Work out the finished part from the listing and answer in its coordinate system (mm). Face numbers are marked on the shaded views. A direction names the side the tool comes from. Round coordinates to 2 decimals unless told otherwise and drop trailing zeros. Loops run counter-clockwise (first coordinate to the right, second up) from the corner with the lowest first, then second, coordinate; pieces in that order, holes last. Notation, with made-up numbers: (-15.5, 24.5) - (12.5, 24.5) arc R22 cw to (12.5, 47.5) - close; hole circle Ø1 at (-16, 49.25). An arc over 180 degrees is marked (long way). Return JSON: item names as keys, results as strings.
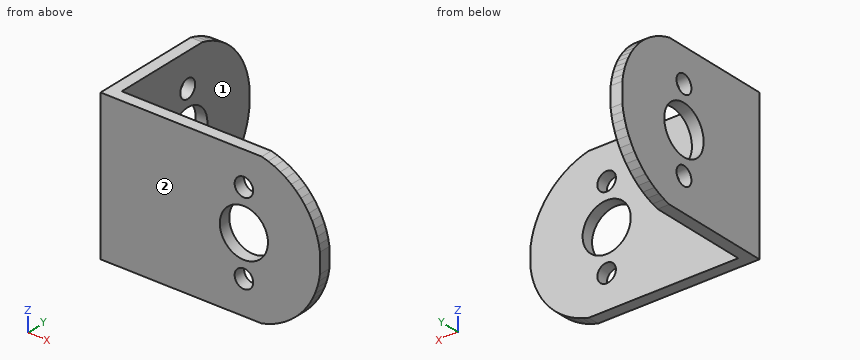
from build123d import *

# Parameters (mm, degrees)
SALIENTE_EXTRUIR1_DEPTH = 2.000000328
CROQUIS2_W              = 2.000000328
CROQUIS2_H              = 25.499995797
SALIENTE_EXTRUIR2_DEPTH = 17.052894691
SALIENTE_EXTRUIR3_DEPTH = 2.000000095
CORTAR_EXTRUIR1_DEPTH   = 92.062133489
CORTAR_EXTRUIR2_DEPTH   = 92.062133489
CORTAR_EXTRUIR3_DEPTH   = 85.413414633
CORTAR_EXTRUIR4_DEPTH   = 85.413414633
CORTAR_EXTRUIR5_DEPTH   = 85.413414633
CORTAR_EXTRUIR6_DEPTH   = 91.256922872
CROQUIS10_R             = 4.160635969
CROQUIS10_R_2           = 1.574242088
CORTAR_EXTRUIR7_DEPTH   = 92.062133489
CROQUIS11_R             = 4.116064073
CROQUIS11_R_2           = 1.582596422
CORTAR_EXTRUIR8_DEPTH   = 86.074229775


with BuildPart() as part:
    # Croquis1 → Saliente-Extruir1 (new body)
    with BuildSketch(Plane(origin=(-18.750000745, 0, 0), x_dir=(0, -1, 0), z_dir=(-1, 0, 0))):
        Polygon((-19.052894786, -77.749997377), (-19.052894786, -52.25000158), (-20.138457417, -52.559908479), (-21.193336695, -52.962061018), (-22.209705785, -53.453475237), (-23.180030286, -54.030507803), (-24.097116664, -54.688870907), (-24.954162538, -55.423695594), (-25.744814426, -56.229524314), (-26.46320872, -57.100389153), (-27.104021981, -58.029823005), (-27.662498876, -59.010945261), (-28.134498745, -60.036472976), (-28.51652354, -61.098802835), (-28.805738315, -62.190063298), (-28.999999166, -63.302159309), (-28.999999166, -66.697835922), (-28.805738315, -67.809939384), (-28.51652354, -68.901196122), (-28.134498745, -69.963529706), (-27.662498876, -70.989057422), (-27.104021981, -71.970179677), (-26.46320872, -72.899609804), (-25.744814426, -73.770478368), (-24.954162538, -74.576310813), (-24.097116664, -75.311124325), (-23.180030286, -75.969494879), (-22.209705785, -76.546527445), (-21.193336695, -77.037930489), (-20.138457417, -77.440083027), align=None)
    extrude(amount=-SALIENTE_EXTRUIR1_DEPTH)

    # Croquis2 → Saliente-Extruir2 (add)
    with BuildSketch(Plane.XZ.offset(-19.052894786)):
        with Locations((-17.750000581, -64.999999479)):
            Rectangle(CROQUIS2_W, CROQUIS2_H)
    extrude(amount=SALIENTE_EXTRUIR2_DEPTH)

    # Croquis3 → Saliente-Extruir3 (add)
    with BuildSketch(Plane.XZ.offset(-2.000000095)):
        Polygon((8.802894503, -77.749997377), (-18.750000745, -77.749997377), (-18.750000745, -52.25000158), (8.802894503, -52.25000158), (9.888458066, -52.559908479), (10.943335481, -52.962061018), (11.959705502, -53.453475237), (12.930030003, -54.030507803), (13.84711545, -54.688870907), (14.704162255, -55.423695594), (15.494815074, -56.229524314), (16.213208437, -57.100389153), (16.854021698, -58.029823005), (17.412498593, -59.010945261), (17.884498462, -60.036472976), (18.266523257, -61.098802835), (18.555738032, -62.190063298), (18.750000745, -63.302159309), (18.750000745, -66.697835922), (18.555738032, -67.809939384), (18.266523257, -68.901196122), (17.884498462, -69.963529706), (17.412498593, -70.989057422), (16.854021698, -71.970179677), (16.213208437, -72.899609804), (15.494815074, -73.770478368), (14.704162255, -74.576310813), (13.84711545, -75.311124325), (12.930030003, -75.969494879), (11.959705502, -76.546527445), (10.943335481, -77.037930489), (9.888458066, -77.440083027), align=None)
    extrude(amount=SALIENTE_EXTRUIR3_DEPTH)

    # Croquis4 → Cortar-Extruir1 (cut, through all)
    with BuildSketch(Plane.ZY.offset(18.750000745)):
        Polygon((-67.884810269, 13.229101896), (-67.402966321, 12.802229263), (-66.858895123, 12.458175421), (-66.266670823, 12.205854058), (-65.641649067, 12.051798403), (-64.999997616, 12.000000104), (-64.358353615, 12.051798403), (-63.733331859, 12.205854058), (-63.141107559, 12.458175421), (-62.597028911, 12.802229263), (-62.115188688, 13.229101896), (-61.708066612, 13.727741316), (-61.386201531, 14.285230078), (-61.157926917, 14.887129888), (-61.029162258, 15.517854132), (-61.003241688, 16.161063686), (-61.08083576, 16.800101846), (-61.259932816, 17.41841808), (-61.535898596, 17.999999225), (-61.901580542, 18.529782072), (-62.347508967, 18.99404265), (-62.86213547, 19.380759448), (-63.432134688, 19.679918885), (-64.04273957, 19.883768633), (-64.678132534, 19.987029955), (-65.321870148, 19.987029955), (-65.957263112, 19.883768633), (-66.567860544, 19.679918885), (-67.137859762, 19.380759448), (-67.652486265, 18.99404265), (-68.098418415, 18.529782072), (-68.464100361, 17.999999225), (-68.740069866, 17.41841808), (-68.919159472, 16.800101846), (-68.996757269, 16.161063686), (-68.970829248, 15.517854132), (-68.842068315, 14.887129888), (-68.613797426, 14.285230078), (-68.291939795, 13.727741316), align=None)
    extrude(amount=-CORTAR_EXTRUIR1_DEPTH, mode=Mode.SUBTRACT)

    # Croquis5 → Cortar-Extruir2 (cut, through all)
    with BuildSketch(Plane.ZY.offset(18.750000745)):
        Polygon((-57.250000536, 14.700962231), (-56.939337403, 14.939339831), (-56.700963527, 15.250000171), (-56.551113725, 15.611771494), (-56.499999017, 16.00000076), (-56.551113725, 16.388230026), (-56.700963527, 16.750000417), (-56.939337403, 17.060659826), (-57.250000536, 17.299037427), (-57.611770928, 17.448889092), (-57.999998331, 17.500000075), (-58.38822946, 17.448889092), (-58.749999851, 17.299037427), (-59.060662985, 17.060659826), (-59.29903686, 16.750000417), (-59.448886663, 16.388230026), (-59.500001371, 16.00000076), (-59.448886663, 15.611771494), (-59.29903686, 15.250000171), (-59.060662985, 14.939339831), (-58.749999851, 14.700962231), (-58.38822946, 14.551111497), (-57.999998331, 14.499999583), (-57.611770928, 14.551111497), align=None)
    extrude(amount=-CORTAR_EXTRUIR2_DEPTH, mode=Mode.SUBTRACT)

    # Croquis6 → Cortar-Extruir3 (cut, through all)
    with BuildSketch(Plane(origin=(0, 2.000000095, 0), x_dir=(-1, 0, 0), z_dir=(0, 1, 0))):
        Polygon((-4.450961947, -57.250000536), (-4.689339548, -56.939337403), (-4.999999888, -56.700963527), (-5.361771677, -56.551113725), (-5.750000011, -56.499999017), (-6.138228346, -56.551113725), (-6.500000134, -56.700963527), (-6.810660474, -56.939337403), (-7.049038075, -57.250000536), (-7.198888808, -57.611770928), (-7.249999791, -57.999998331), (-7.198888808, -58.38822946), (-7.049038075, -58.749999851), (-6.810660474, -59.060662985), (-6.500000134, -59.29903686), (-6.138228346, -59.448886663), (-5.750000011, -59.500001371), (-5.361771677, -59.448886663), (-4.999999888, -59.29903686), (-4.689339548, -59.060662985), (-4.450961947, -58.749999851), (-4.301111214, -58.38822946), (-4.250000231, -57.999998331), (-4.301111214, -57.611770928), align=None)
    extrude(amount=-CORTAR_EXTRUIR3_DEPTH, mode=Mode.SUBTRACT)

    # Croquis7 → Cortar-Extruir4 (cut, through all)
    with BuildSketch(Plane(origin=(0, 2.000000095, 0), x_dir=(-1, 0, 0), z_dir=(0, 1, 0))):
        Polygon((-5.750000011, -73.49999994), (-5.361771677, -73.448888958), (-4.999999888, -73.299042881), (-4.689339548, -73.060661554), (-4.450961947, -72.750002146), (-4.301111214, -72.388231754), (-4.250000231, -71.999996901), (-4.301111214, -71.611769497), (-4.450961947, -71.249999106), (-4.689339548, -70.939339697), (-4.999999888, -70.700958371), (-5.361771677, -70.551112294), (-5.750000011, -70.500001311), (-6.138228346, -70.551112294), (-6.500000134, -70.700958371), (-6.810660474, -70.939339697), (-7.049038075, -71.249999106), (-7.198888808, -71.611769497), (-7.249999791, -71.999996901), (-7.198888808, -72.388231754), (-7.049038075, -72.750002146), (-6.810660474, -73.060661554), (-6.500000134, -73.299042881), (-6.138228346, -73.448888958), align=None)
    extrude(amount=-CORTAR_EXTRUIR4_DEPTH, mode=Mode.SUBTRACT)

    # Croquis8 → Cortar-Extruir5 (cut, through all)
    with BuildSketch(Plane(origin=(0, 2.000000095, 0), x_dir=(-1, 0, 0), z_dir=(0, 1, 0))):
        Polygon((-2.208175836, -63.141107559), (-2.55222898, -62.597028911), (-2.979102544, -62.115188688), (-3.477741033, -61.708066612), (-4.035229795, -61.386201531), (-4.63713007, -61.157926917), (-5.267853383, -61.029162258), (-5.911063869, -61.003241688), (-6.550102495, -61.08083576), (-7.168419193, -61.259932816), (-7.749999873, -61.535898596), (-8.279781789, -61.901580542), (-8.744043298, -62.347508967), (-9.130760096, -62.86213547), (-9.429917671, -63.432134688), (-9.633767419, -64.04273957), (-9.73702874, -64.678132534), (-9.73702874, -65.321870148), (-9.633767419, -65.957263112), (-9.429917671, -66.567860544), (-9.130760096, -67.137859762), (-8.744043298, -67.652486265), (-8.279781789, -68.098418415), (-7.749999873, -68.464100361), (-7.168419193, -68.740069866), (-6.550102495, -68.919159472), (-5.911063869, -68.996757269), (-5.267853383, -68.970829248), (-4.63713007, -68.842068315), (-4.035229795, -68.613797426), (-3.477741033, -68.291939795), (-2.979102544, -67.884810269), (-2.55222898, -67.402966321), (-2.208175836, -66.858895123), (-1.955854241, -66.266670823), (-1.801798935, -65.641649067), (-1.750000054, -64.999997616), (-1.801798935, -64.358353615), (-1.955854241, -63.733331859), align=None)
    extrude(amount=-CORTAR_EXTRUIR5_DEPTH, mode=Mode.SUBTRACT)

    # Croquis9 → Cortar-Extruir6 (cut, through all)
    with BuildSketch(Plane(origin=(-16.750000417, 0, 0), x_dir=(0, 0, -1), z_dir=(1, 0, 0))):
        Polygon((72.750002146, 14.700962231), (73.060661554, 14.939339831), (73.299042881, 15.250000171), (73.448888958, 15.611771494), (73.49999994, 16.00000076), (73.448888958, 16.388230026), (73.299042881, 16.750000417), (73.060661554, 17.060659826), (72.750002146, 17.299037427), (72.388231754, 17.448889092), (71.999996901, 17.500000075), (71.611769497, 17.448889092), (71.249999106, 17.299037427), (70.939339697, 17.060659826), (70.700958371, 16.750000417), (70.551112294, 16.388230026), (70.500001311, 16.00000076), (70.551112294, 15.611771494), (70.700958371, 15.250000171), (70.939339697, 14.939339831), (71.249999106, 14.700962231), (71.611769497, 14.551111497), (71.999996901, 14.499999583), (72.388231754, 14.551111497), align=None)
    extrude(amount=-CORTAR_EXTRUIR6_DEPTH, mode=Mode.SUBTRACT)

    # Croquis10 → Cortar-Extruir7 (cut, through all)
    with BuildSketch(Plane.ZY.offset(18.750000745)):
        with Locations((-65.013688685, 15.96331425)):
            Circle(CROQUIS10_R)
        with Locations((-57.995421153, 15.96331425)):
            Circle(CROQUIS10_R_2)
        with Locations(Location((-72.031956216, 15.96331425, 0), (0, 0, 180))):
            Circle(CROQUIS10_R_2)
    extrude(amount=-CORTAR_EXTRUIR7_DEPTH, mode=Mode.SUBTRACT)

    # Croquis11 → Cortar-Extruir8 (cut, through all)
    with BuildSketch(Plane.XZ):
        with Locations(Location((5.743514397, -64.999997616, 0), (0, 0, 270))):
            Circle(CROQUIS11_R)
        with Locations(Location((5.750000011, -57.999998331, 0), (0, 0, 270))):
            Circle(CROQUIS11_R_2)
        with Locations(Location((5.750000011, -71.999996901, 0), (0, 0, 270))):
            Circle(CROQUIS11_R_2)
    extrude(amount=-CORTAR_EXTRUIR8_DEPTH, mode=Mode.SUBTRACT)


solid = part.part
1) A tool of negligible diameter and unlimited length cuts with its end or side. For the marked faces 1 and 2, from which of +Z, -Z, +X, -X, +Y, -Y can it reach the whole face along a straight path? Write none if from no direction.
Verdict:
{"face 1": "+Z, -Z, +X, +Y", "face 2": "+Z, -Z, +X, -X, -Y"}
2) Section B-B (z = -67.25) is taken. Give the vertices of the cut face in (x, y).
Verdict:
{"outline": "(-18.75, 0) - (2.3, 0) - (2.3, 2) - (-16.75, 2) - (-16.75, 12.45) - (-18.75, 12.45) - close; (-18.75, 19.47) - (-16.75, 19.47) - (-16.75, 28.9) - (-18.75, 28.9) - close; (9.19, 0) - (18.65, 0) - (18.65, 2) - (9.19, 2) - close"}
3) Section A-A (x = 3) is taken. Give the vertices of the cut face in (y, z), and give its area (3 significant figures).
Verdict:
{"outline": "(0, -77.75) - (2, -77.75) - (2, -68.07) - (0, -68.07) - close; (0, -61.93) - (2, -61.93) - (2, -52.25) - (0, -52.25) - close", "area": "38.7 mm2"}
4) Find the intervals of material crossed by L1, parallel to X at y = 25.25, z = -74; L2, parallel to Y at x = 7.5, z = -70.5, in increasing order.
Verdict:
{"L1": "x = -18.75 to -16.75", "L2": "y = 0 to 2"}
5) Flat-ended cylindrical pins translate along their axes: pin 1 (1.9 mm diameter, centred on x = 5.75, z = -72, fed in from -Y); pin 2 (12.5 mm diameter, centred on x = 5.5, z = -59.5, fed in from +Y). Find the tip coordinate at first contact, or state that the pin passes through.
Verdict:
{"pin 1": "passes through", "pin 2": "stops at y = 2"}
6) Section D-D (y = 10.25) is taken. Give the vertices of the cut face in (x, z), and give its area (3 significant figures).
Verdict:
{"outline": "(-18.75, -77.75) - (-16.75, -77.75) - (-16.75, -52.25) - (-18.75, -52.25) - close", "area": "51.0 mm2"}
7) Section C-C (x = -7) is taken. Give the vertices of the cut face in (y, z), and give its area (3 significant figures).
Verdict:
{"outline": "(0, -77.75) - (2, -77.75) - (2, -52.25) - (0, -52.25) - close", "area": "51.0 mm2"}
